```python
from build123d import *

# Parameters (mm, degrees)
F1_DEPTH = 100
F2_T     = -1
F5_D     = 20


# Not quite as in the source:
# - the program builds the solid bodies; features that only make, move or delete a surface that nothing else refers to are left out


with BuildPart() as f1:
    # F0 (on Front) → F1 (new body)
    with BuildSketch(Plane.XZ):
        Polygon((0, 200), (0, 0), (200, 0), (1400, 600), (1600, 600), (1600, 800), (1400, 800), (200, 200), align=None)
    extrude(amount=F1_DEPTH)

    # F2
    f2_openings = [f1.faces().sort_by_distance(p)[0] for p in [
        (100, -50, 200),
        (1500, -50, 800),
        (800, -50, 500),
    ]]
    offset(amount=F2_T, openings=f2_openings, kind=Kind.INTERSECTION)

    # F5 (through all)
    with Locations(Plane.XY.offset(601)):
        with Locations((1587, -13), (1587, -87)):
            Hole(F5_D / 2)


solid = f1.part
```
Check sheet for the modelled part. Datum: model origin and axes. Units: mm. A direction names the side the tool comes from. Round coordinates to 2 decimals unless told otherwise and drop trailing zeros. Loops run counter-clockwise (first coordinate to the right, second up) from the corner with the lowest first, then second, coordinate; pieces in that order, holes last. Notation, with made-up numbers: M 32,-27 L 87,-27 A5 cw 87,-18 Z; hole C 5.5,60.5 d10. An arc over 180 degrees is marked long. Answer as a JSON object with one key per item and string values.
1. Section check C-C (z = 114). Record the boundary of the cut face in (x, y), plus the area to 3 significant figures.
Reply:
{"outline": "M 0,-100 L 428,-100 L 428,0 L 0,0 Z; hole M 1,-99 L 425.76,-99 L 425.76,-1 L 1,-1 Z", "area": "1,170 mm²"}
2. Section check D-D (x = 950). Record the boundary of the cut face in (y, z).
Reply:
{"outline": "M -100,375 L 0,375 L 0,575 L -1,575 L -1,376.12 L -99,376.12 L -99,575 L -100,575 Z"}
3. Section check A-A (z = 697). Record the boundary of the cut face in (x, y).
Reply:
{"outline": "M 1194,-100 L 1600,-100 L 1600,0 L 1194,0 L 1194,-1 L 1599,-1 L 1599,-99 L 1194,-99 Z"}
4. Access from +Z, -Z, +X, -X, +Y, -Y to the whole of each face (thin tool, end or side, straight path). Record for faces 4 (the flat face through (808.4, -0.5, 504.2)), 5 (the flat face through (1599, -49, 699)), 6 (the flat face through (1, -49, 102)), 7 (the flat face through (1499, -49, 600)), 8 (the flat face through (1600, -49, 699)).
Reply:
{"face 4": "+Z, -X, +Y, -Y", "face 5": "+Z, -X", "face 6": "+Z", "face 7": "-Z, +X, +Y, -Y", "face 8": "+Z, -Z, +X, +Y, -Y"}
5. Section check B-B (y = -47). Record the boundary of the cut face in (x, z), plus the area to 3 significant figures.
Reply:
{"outline": "M 0,0 L 200,0 L 1400,600 L 1600,600 L 1600,800 L 1599,800 L 1599,601 L 1399.76,601 L 199.76,1 L 1,1 L 1,200 L 0,200 Z", "area": "2,140 mm²"}
6. Mould release check, pull along X, two halves, no side actions. Record for faces 1 (the flat face through (796, -1, 432)), 2 (the flat face through (796, 0, 431)), 3 (the flat face through (808.4, -99.5, 504.2)): pulls with the +X half, pulls with the -X half, needs draft (parallel to the pull), parting line crosses it, or undercut.
Reply:
{"face 1": "undercut", "face 2": "needs draft", "face 3": "pulls with the -X half"}
7. Scan lines: line 1 (Y direction, x = 1587, z = 600.85); line 2 (Y direction, x = 413, z = 185.5); line 3 (Z direction, x = 148, y = -56). Record each from-to range of solid material in increasing order.
Reply:
{"line 1": "y = -100 to -97, -77 to -23, -3 to 0", "line 2": "y = -100 to -99, -1 to 0", "line 3": "z = 0 to 1"}
8. Gauge pin test, flat ends, axial feed: P1, Ø4, axis at x = 415.5, y = -14, coming from the -Z side; P2, Ø12, axis at x = 841.5, y = -48.5, coming from the +Z side; P3, Ø3, axis at x = 1014, y = -88, coming from the -Z side; P4, Ø16, axis at x = 1587, y = -87, coming from the -Z side. Record the tip position at first contact, or that the pin passes through.
Reply:
{"P1": "stops at z = 106.75", "P2": "stops at z = 324.87", "P3": "stops at z = 406.25", "P4": "passes through"}
